Could you check a few things on this model? Use its own coordinates, in mm. A direction names the side the tool comes from. Round coordinates to 2 decimals unless told otherwise and drop trailing zeros. Write each loop counter-clockwise with the first axis right and the second up, starting at its lowest first coordinate (ties: lowest second). Pieces come first, ordered by that corner, then holes. Notation, with made-up numbers: (57, -38) -> (113, -38) arc R18 ccw to (113, -11) -> close; hole circle Ø10 at (8.5, 73). An arc over 180 degrees is marked (long way). Return JSON: item names as keys, results as strings.
from build123d import *

# Parameters (mm, degrees)
BOSS_EXTRUDE1_DEPTH     = 1
FILLET2_R               = 1
SKETCH3_W               = 10
SKETCH3_H               = 7
BOSS_EXTRUDE2_DEPTH     = 2
SKETCH4_W               = 22.85
SKETCH4_H               = 22.85
BOSS_EXTRUDE3_DEPTH     = 1.3
SKETCH7_W               = 4
SKETCH7_H               = 4
BOSS_EXTRUDE4_DEPTH     = 2.5
FILLET3_R               = 10
FILLET4_R               = 10
TAP_DRILL_FOR_M2_TAP1_D = 1.6
SKETCH11_W              = 22.85
SKETCH11_H              = 1.3
BOSS_EXTRUDE5_DEPTH     = 1
SKETCH12_W              = 1
SKETCH12_H              = 10
SKETCH12_H_2            = 4.85
BOSS_EXTRUDE6_DEPTH     = 3
SKETCH13_R              = 1
BOSS_EXTRUDE7_DEPTH     = 2.5
CHAMFER2_SIZE           = 0.5


with BuildPart() as part:
    # Sketch2 → Boss-Extrude1 (new body)
    with BuildSketch(Plane(origin=(0, 0, 0), x_dir=(0, 1, 0), z_dir=(0, 0, 1))):
        Polygon((-7.2, 11.5), (-7.2, -11.5), (-4.8, -11.5), (-4.8, -10), (4.8, -10), (4.8, -11.5), (7.2, -11.5), (7.2, 11.5), (4.8, 11.5), (4.8, 5.1), (-4.8, 5.1), (-4.8, 11.5), align=None)
    extrude(amount=BOSS_EXTRUDE1_DEPTH)

    # Fillet2
    fillet2_edges = [part.edges().sort_by_distance(p)[0] for p in [
        (11.5, 7.2, 0.5),
        (11.5, 4.8, 0.5),
        (11.5, -4.8, 0.5),
        (11.5, -7.2, 0.5),
        (-11.5, -7.2, 0.5),
        (-11.5, -4.8, 0.5),
        (-11.5, 4.8, 0.5),
        (-11.5, 7.2, 0.5),
    ]]
    fillet(fillet2_edges, radius=FILLET2_R)

    # Sketch3 → Boss-Extrude2 (add)
    with BuildSketch(Plane.XY.offset(1)):
        with Locations((2.45, 0)):
            Rectangle(SKETCH3_W, SKETCH3_H)
    extrude(amount=BOSS_EXTRUDE2_DEPTH)

    # Sketch4 → Boss-Extrude3 (add)
    with BuildSketch(Plane.XY.offset(3)):
        with Locations((2.45, 0)):
            Rectangle(SKETCH4_W, SKETCH4_H)
    extrude(amount=BOSS_EXTRUDE3_DEPTH)

    # Sketch7 → Boss-Extrude4 (add)
    with BuildSketch(Plane.XY.offset(4.3)):
        with Locations((2.45, 13.425)):
            Rectangle(SKETCH7_W, SKETCH7_H)
        with Locations((2.45, -13.425)):
            Rectangle(SKETCH7_W, SKETCH7_H)
    extrude(amount=-BOSS_EXTRUDE4_DEPTH)

    # Fillet3
    # the kernel refuses this fillet: 10 mm, written as the material it adds along each edge
    with BuildSketch(Plane(origin=(0.45, 11.425, 3), x_dir=(0, -1, 0), z_dir=(1, 0, 0))) as fillet3_piece_1:
        with BuildLine():
            CenterArc((4.749736835, 10), FILLET3_R, 241.642363424, 28.357636576)
            Line((0, 1.2), (0, 0))
            Line((0, 0), (4.749736835, 0))
        make_face()
    extrude(amount=4)

    # Fillet4
    # the kernel refuses this fillet: 10 mm, written as the material it adds along each edge
    with BuildSketch(Plane(origin=(4.45, -11.425, 3), x_dir=(0, 1, 0), z_dir=(-1, 0, 0))) as fillet4_piece_1:
        with BuildLine():
            CenterArc((4.749736835, 10), FILLET4_R, 241.642363424, 28.357636576)
            Line((0, 1.2), (0, 0))
            Line((0, 0), (4.749736835, 0))
        make_face()
    extrude(amount=4)

    # Tap Drill for M2 Tap1 (through all)
    with Locations(Plane.XY.offset(4.3)):
        with Locations((2.45, 13.425), (2.45, -13.425)):
            Hole(TAP_DRILL_FOR_M2_TAP1_D / 2)

    # Sketch11 → Boss-Extrude5 (add)
    with BuildSketch(Plane.YZ.offset(13.875)):
        with Locations((0, 3.65)):
            Rectangle(SKETCH11_W, SKETCH11_H)
    extrude(amount=BOSS_EXTRUDE5_DEPTH)

    # Sketch12 → Boss-Extrude6 (add)
    with BuildSketch(Plane.XY.offset(4.3)):
        with Locations((14.375, -6.425)):
            Rectangle(SKETCH12_W, SKETCH12_H)
        with Locations((14.375, 9)):
            Rectangle(SKETCH12_W, SKETCH12_H_2)
    extrude(amount=BOSS_EXTRUDE6_DEPTH)

    # Sketch13 → Boss-Extrude7 (add)
    with BuildSketch(Plane.XY.offset(4.3)):
        with Locations((12.875, 2.505)):
            Circle(SKETCH13_R)
        with Locations((2.45, 4)):
            Circle(SKETCH13_R)
        with Locations((2.45, -4)):
            Circle(SKETCH13_R)
    extrude(amount=BOSS_EXTRUDE7_DEPTH)

    # Chamfer2
    chamfer2_edges = [part.edges().sort_by_distance(p)[0] for p in [
        (11.875, 2.505, 6.8),
        (1.45, -4, 6.8),
        (1.45, 4, 6.8),
    ]]
    chamfer(chamfer2_edges, length=CHAMFER2_SIZE)


solid = part.part
1) I want a section at C-C, the plane z = 5.25. Please give me the cut outline in (x, y) (3 decimals), and give its area (3 significant figures).
Return value:
{"outline": "circle Ø2 at (2.45, -4); circle Ø2 at (2.45, 4); circle Ø2 at (12.875, 2.505); (13.875, -11.425) -> (14.875, -11.425) -> (14.875, -1.425) -> (13.875, -1.425) -> close; (13.875, 6.575) -> (14.875, 6.575) -> (14.875, 11.425) -> (13.875, 11.425) -> close", "area": "24.3 mm²"}
2) I want a section at D-D, the plane x = 2.45. Count the separate pieces of the cut face and the enclosed holes in it, and give its area (3 significant figures).
Return value:
{"separate pieces": "3", "enclosed holes": "0", "area": "83.3 mm²"}
3) I want a section at B-B, the plane x = 8.25. Please give me the cut outline in (y, z) (3 decimals), and give its area (3 significant figures).
Return value:
{"outline": "(-11.425, 3) -> (11.425, 3) -> (11.425, 4.3) -> (-11.425, 4.3) -> close; (-7.2, 0) -> (7.2, 0) -> (7.2, 1) -> (-7.2, 1) -> close", "area": "44.1 mm²"}
4) I want a section at A-A, the plane y = -4. Please give me the cut outline in (x, z) (3 decimals), and give its area (3 significant figures).
Return value:
{"outline": "(-8.975, 3) -> (14.875, 3) -> (14.875, 7.3) -> (13.875, 7.3) -> (13.875, 4.3) -> (3.45, 4.3) -> (3.45, 6.3) -> (2.95, 6.8) -> (1.95, 6.8) -> (1.45, 6.3) -> (1.45, 4.3) -> (-8.975, 4.3) -> close; (-5.1, 0) -> (10, 0) -> (10, 1) -> (-5.1, 1) -> close", "area": "53.9 mm²"}
5) Will these pins go through, and if not, where does the flat tip stop? pin 1 Ø3 at (x, z) = (9, 4) entering from +Y (3 decimals); pin 2 Ø2 at (x, y) = (2.5, 14) entering from -Z; pin 3 Ø6 at (x, y) = (-2, 1) entering from +Z.
Return value:
{"pin 1": "y = 11.425", "pin 2": "z = 1.8", "pin 3": "z = 4.3"}
6) Thinking about a two-plate mould opening in X: for faces 1 (the face through (11.199, 5.085, 0.507)), 2 (the face through (2.4, 4, 6.8)), 3 (the face through (12.66, 1.53, 5.29)), which applies, pulls with the +X half, pulls with the -X half, needs draft (parallel to the pull), parting line crosses it, or undercut?
Return value:
{"face 1": "pulls with the +X half", "face 2": "needs draft", "face 3": "undercut"}
7) For faces 4 (the face through (2.4, -4, 6.8)), 5 (the face through (7.45, 0, 2)), 6 (the face through (11.215, -5.101, 0.507)), 7 (the face through (13.875, -6, 6)), 8 (the face through (-7.8, 4.8, 0.5)), which set-ups out of +Z, -Z, +X, -X, +Y, -Y let a thin tool reach every point of the face, with its end or its side?
Return value:
{"face 4": "+Z, -X, +Y, -Y", "face 5": "+X, +Y, -Y", "face 6": "-Z, +X", "face 7": "+Z, -Y", "face 8": "-Z, -X"}
8) If I drill on probe 1 along Z at (x, y) = (3.5, -6); probe 2 along Y at (x, z) = (2.45, 3.65) (3 decimals); probe 3 along Y at (x, z) = (2, 3.5) (3 decimals), over which ranges is the centre line in solid material (lowest first)? Write a range as [from, to].
Return value:
{"probe 1": "[0, 1], [3, 4.3]", "probe 2": "[-15.425, -14.225], [-12.625, 12.625], [14.225, 15.425]", "probe 3": "[-15.425, -14.086], [-12.764, 12.764], [14.086, 15.425]"}
